Read the model definition and answer for the solid it produces. Units are mm, in the model's axes. A direction names the side the tool comes from. Coordinates: 2 decimals unless noted, no trailing zeros. Loops run counter-clockwise (first coordinate to the right, second up) from the corner with the lowest first, then second, coordinate; pieces in that order, holes last. Notation, with made-up numbers: (49, 27.25) - (77, 27.25) arc R28 ccw to (77, 53.25) - close; hole circle Ø10 at (-35.75, -32.5). An arc over 180 degrees is marked (long way). Use one line per item in the form item = value.
from build123d import *

# Parameters (mm, degrees)
SKETCH_1_W                        = 646.5
SKETCH_1_H                        = 540
SKETCH_1_R                        = 3
SM_BASE_FLANGE_1_DEPTH            = 0.8
SM_EDGE_FLANGE_1_STRIP_W          = 4.2
SM_EDGE_FLANGE_1_STRIP_H          = 0.8
SM_EDGE_FLANGE_1_STRIP_CUT_DEPTH  = 440
SM_EDGE_FLANGE_1_RELIEF_W         = 5
SM_EDGE_FLANGE_1_RELIEF_H         = 0.8
SM_EDGE_FLANGE_1_RELIEF_CUT_DEPTH = 0.8
SM_EDGE_FLANGE_1_DEPTH            = 440
SM_EDGE_FLANGE_2_STRIP_W          = 4.2
SM_EDGE_FLANGE_2_STRIP_H          = 0.8
SM_EDGE_FLANGE_2_STRIP_CUT_DEPTH  = 440
SM_EDGE_FLANGE_2_RELIEF_W         = 5
SM_EDGE_FLANGE_2_RELIEF_H         = 0.8
SM_EDGE_FLANGE_2_RELIEF_CUT_DEPTH = 0.8
SM_EDGE_FLANGE_2_DEPTH            = 440
SM_EDGE_FLANGE_3_STRIP_W          = 4.2
SM_EDGE_FLANGE_3_STRIP_H          = 0.8
SM_EDGE_FLANGE_3_STRIP_CUT_DEPTH  = 546.5
SM_EDGE_FLANGE_3_RELIEF_W         = 5
SM_EDGE_FLANGE_3_RELIEF_H         = 0.8
SM_EDGE_FLANGE_3_RELIEF_CUT_DEPTH = 0.8
SM_EDGE_FLANGE_3_DEPTH            = 546.5
SM_EDGE_FLANGE_3_FLAT_DEPTH       = 0.8
SM_EDGE_FLANGE_4_STRIP_W          = 4.2
SM_EDGE_FLANGE_4_STRIP_H          = 0.8
SM_EDGE_FLANGE_4_STRIP_CUT_DEPTH  = 546.5
SM_EDGE_FLANGE_4_RELIEF_W         = 5
SM_EDGE_FLANGE_4_RELIEF_H         = 0.8
SM_EDGE_FLANGE_4_RELIEF_CUT_DEPTH = 0.8
SM_EDGE_FLANGE_4_DEPTH            = 546.5
SM_EDGE_FLANGE_4_FLAT_DEPTH       = 0.8
SKETCH_18_W                       = 85
SKETCH_18_H                       = 42.323448133
CUT_EXTRUDE_1_DEPTH               = 629.964102712
SKETCH_19_W                       = 85
SKETCH_19_H                       = 50.946353984
CUT_EXTRUDE_2_DEPTH               = 629.964102712
SKETCH_20_R                       = 3.5
CUT_EXTRUDE_3_DEPTH               = 630.650063527


# Sheet-metal steps are written as plain solids
with BuildPart() as part:
    # Sketch 1 → 基体-法兰1 (new body)
    with BuildSketch(Plane.XY):
        Rectangle(SKETCH_1_W, SKETCH_1_H)
        with Locations((313.25, 260)):
            Circle(SKETCH_1_R, mode=Mode.SUBTRACT)
        with Locations((-313.25, 260)):
            Circle(SKETCH_1_R, mode=Mode.SUBTRACT)
        with Locations((-313.25, -260)):
            Circle(SKETCH_1_R, mode=Mode.SUBTRACT)
        with Locations((313.25, -260)):
            Circle(SKETCH_1_R, mode=Mode.SUBTRACT)
    extrude(amount=-SM_BASE_FLANGE_1_DEPTH)

    # 边线-法兰1 strip (across the edge) → 边线-法兰1 strip cut (cut)
    with BuildSketch(Plane(origin=(323.25, -220, 0), x_dir=(-1, 0, 0), z_dir=(0, 1, 0))):
        with Locations((-0.8, -0.4)):
            Rectangle(SM_EDGE_FLANGE_1_STRIP_W, SM_EDGE_FLANGE_1_STRIP_H)
    extrude(amount=SM_EDGE_FLANGE_1_STRIP_CUT_DEPTH, mode=Mode.SUBTRACT)

    # 边线-法兰1 relief (on the sheet) → 边线-法兰1 relief cut (cut)
    with BuildSketch(Plane(origin=(321.95, -220, 0), x_dir=(-1, 0, 0), z_dir=(0, 0, 1))):
        with Locations((-1.7, 0.4)):
            Rectangle(SM_EDGE_FLANGE_1_RELIEF_W, SM_EDGE_FLANGE_1_RELIEF_H)
        with Locations((-1.7, -440.4)):
            Rectangle(SM_EDGE_FLANGE_1_RELIEF_W, SM_EDGE_FLANGE_1_RELIEF_H)
    extrude(amount=-SM_EDGE_FLANGE_1_RELIEF_CUT_DEPTH, mode=Mode.SUBTRACT)

    # 边线-法兰1 section (across the edge) → 边线-法兰1 (add)
    with BuildSketch(Plane(origin=(323.25, -220, 0), x_dir=(-1, 0, 0), z_dir=(0, 1, 0))):
        with BuildLine():
            Line((0, 0.5), (0, 19.2))
            Line((0, 19.2), (0.8, 19.2))
            Line((0.8, 19.2), (0.8, 0.5))
            ThreePointArc((0.8, 0.5), (0.946446609, 0.146446609), (1.3, 0))
            Line((1.3, 0), (1.3, -0.8))
            ThreePointArc((1.3, -0.8), (0.380761184, -0.419238816), (0, 0.5))
        make_face()
    extrude(amount=SM_EDGE_FLANGE_1_DEPTH)

    # 边线-法兰2 strip (across the edge) → 边线-法兰2 strip cut (cut)
    with BuildSketch(Plane(origin=(-323.25, 220, 0), x_dir=(1, 0, 0), z_dir=(0, -1, 0))):
        with Locations((-0.8, -0.4)):
            Rectangle(SM_EDGE_FLANGE_2_STRIP_W, SM_EDGE_FLANGE_2_STRIP_H)
    extrude(amount=SM_EDGE_FLANGE_2_STRIP_CUT_DEPTH, mode=Mode.SUBTRACT)

    # 边线-法兰2 relief (on the sheet) → 边线-法兰2 relief cut (cut)
    with BuildSketch(Plane(origin=(-321.95, 220, 0), x_dir=(1, 0, 0), z_dir=(0, 0, 1))):
        with Locations((-1.7, 0.4)):
            Rectangle(SM_EDGE_FLANGE_2_RELIEF_W, SM_EDGE_FLANGE_2_RELIEF_H)
        with Locations((-1.7, -440.4)):
            Rectangle(SM_EDGE_FLANGE_2_RELIEF_W, SM_EDGE_FLANGE_2_RELIEF_H)
    extrude(amount=-SM_EDGE_FLANGE_2_RELIEF_CUT_DEPTH, mode=Mode.SUBTRACT)

    # 边线-法兰2 section (across the edge) → 边线-法兰2 (add)
    with BuildSketch(Plane(origin=(-323.25, 220, 0), x_dir=(1, 0, 0), z_dir=(0, -1, 0))):
        with BuildLine():
            Line((0, 0.5), (0, 19.2))
            Line((0, 19.2), (0.8, 19.2))
            Line((0.8, 19.2), (0.8, 0.5))
            ThreePointArc((0.8, 0.5), (0.946446609, 0.146446609), (1.3, 0))
            Line((1.3, 0), (1.3, -0.8))
            ThreePointArc((1.3, -0.8), (0.380761184, -0.419238816), (0, 0.5))
        make_face()
    extrude(amount=SM_EDGE_FLANGE_2_DEPTH)

    # 边线-法兰3 strip (across the edge) → 边线-法兰3 strip cut (cut)
    with BuildSketch(Plane(origin=(-273.25, -270, 0), x_dir=(0, 1, 0), z_dir=(1, 0, 0))):
        with Locations((-0.8, -0.4)):
            Rectangle(SM_EDGE_FLANGE_3_STRIP_W, SM_EDGE_FLANGE_3_STRIP_H)
    extrude(amount=SM_EDGE_FLANGE_3_STRIP_CUT_DEPTH, mode=Mode.SUBTRACT)

    # 边线-法兰3 relief (on the sheet) → 边线-法兰3 relief cut (cut)
    with BuildSketch(Plane(origin=(-273.25, -268.7, 0), x_dir=(0, 1, 0), z_dir=(0, 0, 1))):
        with Locations((-1.7, 0.4)):
            Rectangle(SM_EDGE_FLANGE_3_RELIEF_W, SM_EDGE_FLANGE_3_RELIEF_H)
        with Locations((-1.7, -546.9)):
            Rectangle(SM_EDGE_FLANGE_3_RELIEF_W, SM_EDGE_FLANGE_3_RELIEF_H)
    extrude(amount=-SM_EDGE_FLANGE_3_RELIEF_CUT_DEPTH, mode=Mode.SUBTRACT)

    # 边线-法兰3 bend section (across the edge) → 边线-法兰3 (add)
    with BuildSketch(Plane(origin=(-273.25, -270, 0), x_dir=(0, 1, 0), z_dir=(1, 0, 0))):
        with BuildLine():
            Line((0, 0.5), (0.8, 0.5))
            ThreePointArc((0.8, 0.5), (0.946446609, 0.146446609), (1.3, 0))
            Line((1.3, 0), (1.3, -0.8))
            ThreePointArc((1.3, -0.8), (0.380761184, -0.419238816), (0, 0.5))
        make_face()
    extrude(amount=SM_EDGE_FLANGE_3_DEPTH)

    # 边线-法兰3 profile (on flange) → 边线-法兰3 flat (add)
    with BuildSketch(Plane.XZ.offset(270)):
        Polygon((-273.25, 0.5), (273.25, 0.5), (273.25, 4.2), (218.25, 4.2), (218.25, 19.2), (-218.25, 19.2), (-218.25, 4.2), (-273.25, 4.2), align=None)
    extrude(amount=-SM_EDGE_FLANGE_3_FLAT_DEPTH)

    # 边线-法兰4 strip (across the edge) → 边线-法兰4 strip cut (cut)
    with BuildSketch(Plane(origin=(273.25, 270, 0), x_dir=(0, -1, 0), z_dir=(-1, 0, 0))):
        with Locations((-0.8, -0.4)):
            Rectangle(SM_EDGE_FLANGE_4_STRIP_W, SM_EDGE_FLANGE_4_STRIP_H)
    extrude(amount=SM_EDGE_FLANGE_4_STRIP_CUT_DEPTH, mode=Mode.SUBTRACT)

    # 边线-法兰4 relief (on the sheet) → 边线-法兰4 relief cut (cut)
    with BuildSketch(Plane(origin=(273.25, 268.7, 0), x_dir=(0, -1, 0), z_dir=(0, 0, 1))):
        with Locations((-1.7, 0.4)):
            Rectangle(SM_EDGE_FLANGE_4_RELIEF_W, SM_EDGE_FLANGE_4_RELIEF_H)
        with Locations((-1.7, -546.9)):
            Rectangle(SM_EDGE_FLANGE_4_RELIEF_W, SM_EDGE_FLANGE_4_RELIEF_H)
    extrude(amount=-SM_EDGE_FLANGE_4_RELIEF_CUT_DEPTH, mode=Mode.SUBTRACT)

    # 边线-法兰4 bend section (across the edge) → 边线-法兰4 (add)
    with BuildSketch(Plane(origin=(273.25, 270, 0), x_dir=(0, -1, 0), z_dir=(-1, 0, 0))):
        with BuildLine():
            Line((0, 0.5), (0.8, 0.5))
            ThreePointArc((0.8, 0.5), (0.946446609, 0.146446609), (1.3, 0))
            Line((1.3, 0), (1.3, -0.8))
            ThreePointArc((1.3, -0.8), (0.380761184, -0.419238816), (0, 0.5))
        make_face()
    extrude(amount=SM_EDGE_FLANGE_4_DEPTH)

    # 边线-法兰4 profile (on flange) → 边线-法兰4 flat (add)
    with BuildSketch(Plane(origin=(0, 270, 0), x_dir=(-1, 0, 0), z_dir=(0, 1, 0))):
        Polygon((-273.25, 0.5), (273.25, 0.5), (273.25, 4.2), (218.25, 4.2), (218.25, 19.2), (-218.25, 19.2), (-218.25, 4.2), (-273.25, 4.2), align=None)
    extrude(amount=-SM_EDGE_FLANGE_4_FLAT_DEPTH)

    # 草图18 → 切除-拉伸1 (cut, through all)
    with BuildSketch(Plane(origin=(0, -269.2, 0), x_dir=(1, 0, 0), z_dir=(0, 1, 0))):
        with Locations((-81.712681962, -21.161724066)):
            Rectangle(SKETCH_18_W, SKETCH_18_H)
    extrude(amount=-CUT_EXTRUDE_1_DEPTH, mode=Mode.SUBTRACT)

    # 草图19 → 切除-拉伸2 (cut, through all)
    with BuildSketch(Plane.XZ.offset(-269.2)):
        with Locations((-81.712681962, 25.473176992)):
            Rectangle(SKETCH_19_W, SKETCH_19_H)
    extrude(amount=-CUT_EXTRUDE_2_DEPTH, mode=Mode.SUBTRACT)

    # 草图20 → 切除-拉伸3 (cut, through all)
    with BuildSketch(Plane(origin=(0, -270, 0), x_dir=(-1, 0, 0), z_dir=(0, -1, 0))):
        with Locations(Location((5.25, -9.2, 0), (0, 0, 90))):
            Circle(SKETCH_20_R)
    extrude(amount=-CUT_EXTRUDE_3_DEPTH, mode=Mode.SUBTRACT)


solid = part.part
Item 1: The part is cut by section D-D on x = -96.5. Give the vertices of the cut face in (y, z), plus the area to 3 significant figures.
Results below:
outline = (-269.9, 0) arc R1.3 ccw to (-268.7, -0.8) - (268.7, -0.8) arc R1.3 ccw to (269.9, 0) - (269.2, 0) - (269.2, 0.5) arc R0.5 cw to (268.7, 0) - (-268.7, 0) arc R0.5 cw to (-269.2, 0.5) - (-269.2, 0) - close
area = 431 mm²
Item 2: Which of the six approach directions +Z, -Z, +X, -X, +Y, -Y give full straight-line access (tool end or side, diameter ignored) to faces 1 (the flat face through (-323.25, 3, 10)), 2 (the flat face through (322.45, -3, 10)), 3 (the flat face through (-181, 269.2, 10))?
Results below:
face_1 = +Z, -Z, -X, +Y, -Y
face_2 = +Z, +Y, -Y
face_3 = +Z, +X, -X
Item 3: The part is cut by section A-A on z = 9.2. Count the separate pieces of the cut face and the enclosed holes in it, plus the area to 3 significant figures.
Results below:
separate_pieces = 8
enclosed_holes = 0
area = 1,260 mm²
Item 4: The part is cut by section B-B on x = -231. Give the vertices of the cut face in (y, z).
Results below:
outline = (-270, 0.5) arc R1.3 ccw to (-268.7, -0.8) - (268.7, -0.8) arc R1.3 ccw to (270, 0.5) - (270, 4.2) - (269.2, 4.2) - (269.2, 0.5) arc R0.5 cw to (268.7, 0) - (-268.7, 0) arc R0.5 cw to (-269.2, 0.5) - (-269.2, 4.2) - (-270, 4.2) - close
Item 5: The part is cut by section C-C on y = -73. Give the vertices of the cut face in (x, z), plus the area to 3 significant figures.
Results below:
outline = (-323.25, 0.5) arc R1.3 ccw to (-321.95, -0.8) - (321.95, -0.8) arc R1.3 ccw to (323.25, 0.5) - (323.25, 19.2) - (322.45, 19.2) - (322.45, 0.5) arc R0.5 cw to (321.95, 0) - (-321.95, 0) arc R0.5 cw to (-322.45, 0.5) - (-322.45, 19.2) - (-323.25, 19.2) - close
area = 547 mm²
Item 6: For a pull along Y with two mould halves and no side action, classify faces 4 (the flat face through (80, -270, 10)), 5 (the flat face through (-5, 4, 0)), 6 (the flat face through (-5, 4, -0.8)), 7 (the flat face through (84, 269.2, 10)) as +Y half, -Y half, draft (parallel to the pull), parting line (faces both ways), or undercut.
Results below:
face_4 = -Y half
face_5 = undercut
face_6 = draft
face_7 = undercut
Item 7: Each of these flat-tipped pins is pushed along its axis until it touches: P1, Ø0.6, axis at y = -269.5, z = 13, coming from the -X side; P2, Ø6, axis at x = -248, y = 144, coming from the +Z side; P3, Ø1.1, axis at x = -322, z = 8.5, coming from the -Y side. Where does it stop, or does it pass through?
Results below:
P1 = -218.25
P2 = 0
P3 = -220
Item 8: Find the intervals of material crossed by L1, parallel to X at y = 260, z = -0.55; L2, parallel to Y at x = -313.25, z = -0.45; L3, parallel to X at y = 269.5, z = 9.2, in increasing order.
Results below:
L1 = -323.25 to -316.25, -310.25 to 310.25, 316.25 to 323.25
L2 = -270 to -263, -257 to 257, 263 to 270
L3 = -218.25 to -124.21, -39.21 to -8.75, -1.75 to 218.25
